Can you work these out from the drawing? Everything is in mm from the part's minimum corner. A direction names the side the tool comes from. Give positions to 0.01 mm unless a question says otherwise; leave off trailing zeros. Loops run counter-clockwise (first coordinate to the right, second up) from the corner with the lowest first, then second, coordinate; pieces in that order, holes last. Notation, with made-up numbers: (-5, 79.25) -> (10, 79.25) arc R28 ccw to (10, 100.25) -> close; hole circle Ø7 at (-22, 24.5). An arc over 180 degrees is marked (long way). Return JSON: item names as keys, results as strings. Group by question number.
Q1. Thinking about a two-plate mould opening in X: for the marked faces 1 and 2, which applies, pulls with the +X half, pulls with the -X half, needs draft (parallel to the pull), parting line crosses it, or undercut?
Q2. Suppose I cut it at B-B, the plane z = 20.25. Please give me the cut outline in (x, y) (1 decimal), and give its area (4 significant figures).
Q3. Will these pins go through, and if not, where does the flat tip stop? pin 1 (8 mm diameter, centred on y = 56.5, z = 12, fed in from +X); pin 2 (2 mm diameter, centred on x = 13, z = 11.5, fed in from -Y); pin 3 (17.5 mm diameter, centred on x = 35.37, y = 35.37, fed in from -Z); pin 4 (1 mm diameter, centred on x = 11.5, z = 18, fed in from -Y).
Q4. Which directions (+Z, -Z, +X, -X, +Y, -Y) give clear straight access to the entire face, cutting with the end or side of a thin tool? Please do the marked faces 3 and 4.
Q5. I need wall thicknesses on line 1 along Y through (x, z) = (33, 2) (1 decimal); line 2 along Z through (x, y) = (26, 39.5); line 3 along Y through (x, z) = (31.5, 6.5) (1 decimal). Which ranges of each line are inside material? Lowest first, please. Write a range as [from, to].
Q6. Suppose I cut it at A-A, the plane z = 14.5. Please give me the cut outline in (x, y), and give its area (3 significant figures).
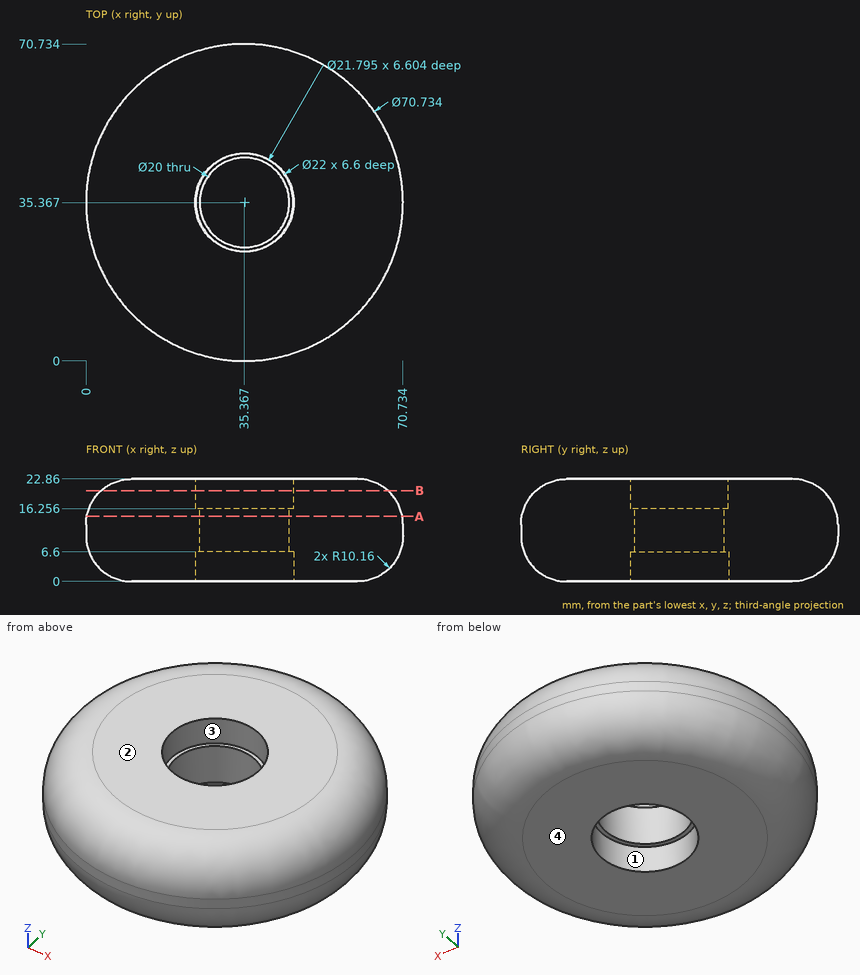
Ans:
{
 "1": {"face 1": "undercut", "face 2": "needs draft"},
 "2": {"outline": "circle Ø64 at (35.4, 35.4); hole circle Ø21.8 at (35.4, 35.4)", "area": "2,845 mm^2"},
 "3": {"pin 1": "stops at x = 66.31", "pin 2": "stops at y = 7.18", "pin 3": "passes through", "pin 4": "stops at y = 10.69"},
 "4": {"face 3": "+Z", "face 4": "-Z, +X, -X, +Y, -Y"},
 "5": {"line 1": "y = [4.2, 24.6], [46.1, 66.5]", "line 2": "z = [6.6, 16.26]", "line 3": "y = [0.9, 25.1], [45.7, 69.8]"},
 "6": {"outline": "circle Ø70.41 at (35.37, 35.37); hole circle Ø20 at (35.37, 35.37)", "area": "3,580 mm^2"}
}
